Check sheet for the modelled part. Datum: model origin and axes. Units: mm. Face numbers are marked on the shaded views. A direction names the side the tool comes from. Give positions to 0.01 mm unless a question says otherwise; leave off trailing zeros. Order: outer loops, then holes, each group sorted by start corner. A loop starts at its lowest first (then second) coordinate and runs counter-clockwise, first axis right, second up. Notation, with made-up numbers: (9.25, -35.5) - (62.25, -35.5) arc R26 ccw to (62.25, -21.5) - close; hole circle Ø9 at (53.5, -33). An arc over 180 degrees is marked (long way). Answer in a Markdown table with one row per item.
from build123d import *

# Parameters (mm, degrees)
F1_DEPTH = 82.55
F2_R     = 3.69316
F3_R     = 1.98374
F4_R     = 1.35255
F4_R_2   = 1.8288
F5_DEPTH = 1.70942
F6_R     = 0.762


with BuildPart() as f1:
    # F0 (on Top) → F1 (new body)
    with BuildSketch(Plane.XY):
        Polygon((0, -13.290575), (0, 0), (-16.70942, 0), (-16.70942, -1.70942), (-1.70942, -1.70942), (-1.70942, -14.999995), (59.49058, -14.999995), (59.49058, -1.70942), (74.49058, -1.70942), (74.49058, 0), (57.78116, 0), (57.78116, -13.290575), align=None)
    extrude(amount=F1_DEPTH)

    # F2
    f2_edges = [f1.edges().sort_by_distance(p)[0] for p in [
        (59.49058, -14.999995, 41.275),
        (-1.70942, -14.999995, 41.275),
        (0, 0, 41.275),
        (57.78116, 0, 41.275),
    ]]
    fillet(f2_edges, radius=F2_R)

    # F3
    f3_edges = [f1.edges().sort_by_distance(p)[0] for p in [
        (0, -13.290575, 41.275),
        (57.78116, -13.290575, 41.275),
        (59.49058, -1.70942, 41.275),
        (-1.70942, -1.70942, 41.275),
    ]]
    fillet(f3_edges, radius=F3_R)

    # F4 (on face) → F5 (cut, through all)
    with BuildSketch(Plane.XZ.offset(14.999995)):
        with Locations((51.82867, 78.58125)):
            Circle(F4_R)
        with Locations((5.95249, 78.58125)):
            Circle(F4_R)
        with Locations((5.95249, 3.96875)):
            Circle(F4_R)
        with Locations((51.82867, 3.96875)):
            Circle(F4_R)
        with Locations((22.08338, 37.30625)):
            Circle(F4_R_2)
        with Locations((22.08338, 45.24375)):
            Circle(F4_R_2)
    extrude(amount=-F5_DEPTH, mode=Mode.SUBTRACT)

    # F6
    f6_edges = [f1.edges().sort_by_distance(p)[0] for p in [
        (-16.70942, -0.85471, 82.55),
        (-16.70942, -0.85471, 0),
        (74.49058, -0.85471, 0),
        (74.49058, -0.85471, 82.55),
    ]]
    fillet(f6_edges, radius=F6_R)


solid = f1.part
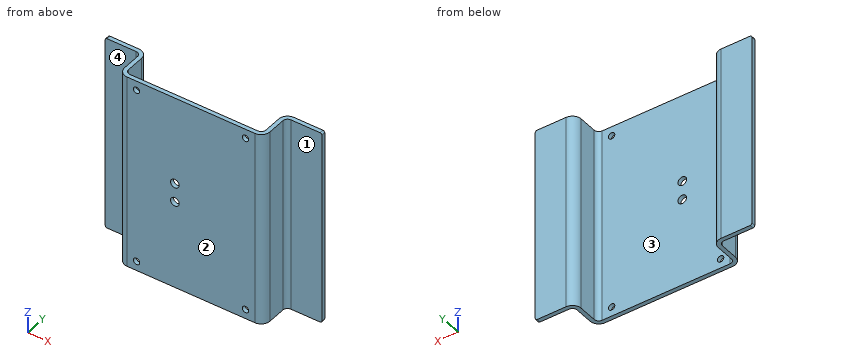
(1) Access from +Z, -Z, +X, -X, +Y, -Y to the whole of each face (thin tool, end or side, straight path). Record for the marked faces 1 and 2.
Geometry says:
| item | result |
|---|---|
| face 1 | +Z, -Z, +X, -Y |
| face 2 | +Z, -Z, +X, -X, -Y |
(2) Mould release check, pull along X, two halves, no side actions. Record for the marked faces 3 and 4: pulls with the +X half, pulls with the -X half, needs draft (parallel to the pull), parting line crosses it, or undercut.
Geometry says:
| item | result |
|---|---|
| face 3 | undercut |
| face 4 | needs draft |
(3) Cross-section at C-C, the plane x = -9. Record the cut outline in (y, z), then the cut area to 3 significant figures.
Geometry says:
| item | result |
|---|---|
| outline | (-1.71, 0) - (0, 0) - (0, 82.55) - (-1.71, 82.55) - close |
| area | 141 mm² |
(4) Thickness scan on L1, parallel to X at y = -6.25, z = 45; L2, parallel to Z at x = 20.5, y = -13.75; L3, parallel to Y at x = -11, z = 34. Record the ranges inside material, lowest first.
Geometry says:
| item | result |
|---|---|
| L1 | -1.71 to 0, 57.78 to 59.49 |
| L2 | 0 to 36.39, 38.22 to 44.33, 46.16 to 82.55 |
| L3 | -1.71 to 0 |
(5) Cross-section at A-A, the plane y = -7.75. Record the cut outline in (x, z).
Geometry says:
| item | result |
|---|---|
| outline | (-1.71, 0) - (0, 0) - (0, 82.55) - (-1.71, 82.55) - close; (57.78, 0) - (59.49, 0) - (59.49, 82.55) - (57.78, 82.55) - close |
(6) Cross-section at B-B, the plane z = 29. Record the cut outline in (x, y), then the cut area to 3 significant figures.
Geometry says:
| item | result |
|---|---|
| outline | (-16.71, -1.71) - (-3.69, -1.71) arc R1.98 cw to (-1.71, -3.69) - (-1.71, -11.31) arc R3.69 ccw to (1.98, -15) - (55.8, -15) arc R3.69 ccw to (59.49, -11.31) - (59.49, -3.69) arc R1.98 cw to (61.47, -1.71) - (74.49, -1.71) - (74.49, 0) - (61.47, 0) arc R3.69 ccw to (57.78, -3.69) - (57.78, -11.31) arc R1.98 cw to (55.8, -13.29) - (1.98, -13.29) arc R1.98 cw to (0, -11.31) - (0, -3.69) arc R3.69 ccw to (-3.69, 0) - (-16.71, 0) - close |
| area | 193 mm² |
(7) Gauge pin test, flat ends, axial feed: P1, Ø6, axis at y = -13, z = 11.5, coming from the -X side; P2, Ø1.6, axis at x = 51.83, z = 78.58, coming from the -Y side; P3, Ø10.5, axis at x = 69, z = 49.5, coming from the -Y side; P4, Ø8.5, axis at y = -6.5, z = 22.5, coming from the -X side. Record the tip position at first contact, or that the pin passes through.
Geometry says:
| item | result |
|---|---|
| P1 | x = -1.71 |
| P2 | through |
| P3 | y = -1.71 |
| P4 | x = -2.33 |
